Part print with two shaded views. Sizes in mm from the minimum x, y, z corner. A direction names the side the tool comes from. Coordinates: 2 decimals unless noted, no trailing zeros. Loops run counter-clockwise (first coordinate to the right, second up) from the corner with the lowest first, then second, coordinate; pieces in that order, holes last.
(1) Slice it at A-A (y = 2.5). Give the cut face in (x, z).
(2) Slice it at C-C (x = 2.85). Give the cut face in (y, z).
(3) Two-plate mould, pull along X, no slides. Class the marked faces 3, 4, 5 and 6: pulls with the +X half, pulls with the -X half, needs draft (parallel to the pull), parting line crosses it, or undercut.
(4) Flat gauge pins, fed straight in: P1, Ø1, axis at y = 1, z = 3.5, coming from the +X side; P2, Ø0.8, axis at x = 2, z = 3, coming from the -Y side. Where does each tip first touch, or does it go through?
(5) Tool access for the marked faces 1 and 2: list every direction of +Z, -Z, +X, -X, +Y, -Y with a clear straight run to the whole face (end or side of a thin tool).
(6) Wall check: L1, parallel to X at y = 3.5, z = 3.6; L2, parallel to Y at x = 1.9, z = 1; L3, parallel to Y at x = 2.8, z = 3.75 (1 decimal). Give the ranges that are in metal, low to high.
(7) Slice it at D-D (x = 0.6). Give the cut face in (y, z).
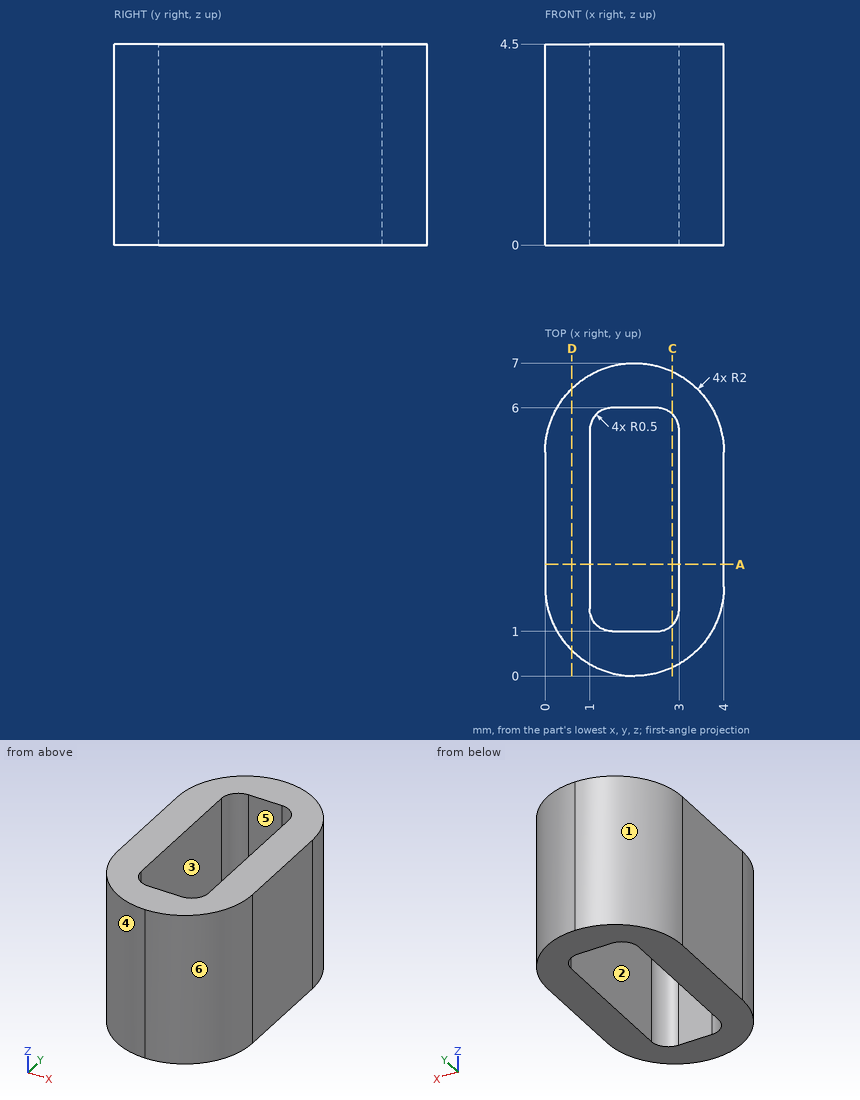
Response values:
1. outline: (0, 0) - (1, 0) - (1, 4.5) - (0, 4.5) - close; (3, 0) - (4, 0) - (4, 4.5) - (3, 4.5) - close
2. outline: (0.19, 0) - (1.14, 0) - (1.14, 4.5) - (0.19, 4.5) - close; (5.86, 0) - (6.81, 0) - (6.81, 4.5) - (5.86, 4.5) - close
3. face 3: undercut
3. face 4: pulls with the -X half
3. face 5: undercut
3. face 6: pulls with the +X half
4. P1: stops at x = 3.94
4. P2: stops at y = 0
5. face 1: +Z, -Z, -X, +Y
5. face 2: +Z, -Z
6. L1: x = 0 to 1, 3 to 4
6. L2: y = 0 to 1, 6 to 7
6. L3: y = 0.2 to 1.1, 5.9 to 6.8
7. outline: (0.57, 0) - (6.43, 0) - (6.43, 4.5) - (0.57, 4.5) - close
